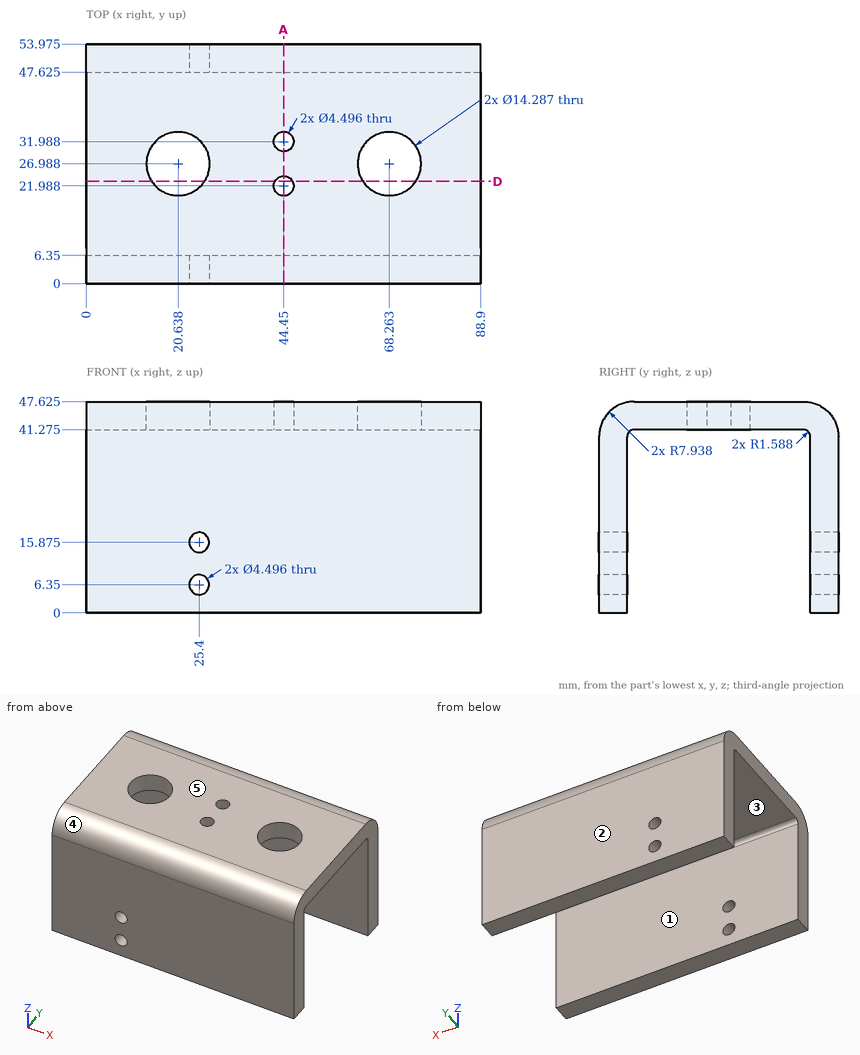
The drawing under review shows one solid part. Ordinate dimensions are in mm from its lowest x, y, z. A direction names the side the tool comes from. Give positions to 0.01 mm unless a question says otherwise; leave off trailing zeros. Write each loop counter-clockwise with the first axis right and the second up, starting at its lowest first coordinate (ties: lowest second). Pieces come first, ordered by that corner, then holes. Notation, with made-up numbers: M -5,71 L 46,71 A23 ccw 46,88 Z; hole C -10,21 d2. An arc over 180 degrees is marked long. Write each question's results on one line, items separated by ' | '. Start each with the question number.
1. Mouldability with a two-part tool opening along Y and no side actions: class the marked faces 3, 4 and 5 as released by +Y, released by -Y, zero draft, split by the parting line, or undercut.
2. We need section D-D (y = 23). Write out the cut boundary in (x, z) (1 decimal).
3. For the marked faces 1 and 2, list the 3-axis set-ups (+Z, -Z, +X, -X, +Y, -Y) from which the entire face can be reached by the end or side of a thin tool; tool diameter is ignored.
4. For probe 1 along Z at (x, y) = (25.4, 1.75) (1 decimal); probe 2 along Z at (x, y) = (25.4, 52.5) (1 decimal); probe 3 along Z at (x, y) = (9, 38.5) (1 decimal), list the stretches that pass through material, from the lowest coordinate up. Write a range as [from, to].
5. We need section A-A (x = 44.45). Count the separate pieces of the cut face and the enclosed holes in it, and give its area (3 significant figures).
6. Insertion check: pin 1 Ø2 at (x, y) = (26.5, 11.5) entering from -Z (1 decimal). The pin has a flat end and moves straight along its axis. Give the tip position at first contact, or say it passes through.
Results found:
1) face 3: undercut | face 4: released by -Y | face 5: zero draft
2) outline: M 0,41.3 L 14.7,41.3 L 14.7,47.6 L 0,47.6 Z; M 26.6,41.3 L 42.4,41.3 L 42.4,47.6 L 26.6,47.6 Z; M 46.5,41.3 L 62.3,41.3 L 62.3,47.6 L 46.5,47.6 Z; M 74.2,41.3 L 88.9,41.3 L 88.9,47.6 L 74.2,47.6 Z
3) face 1: -Z, +X, -X | face 2: +Z, -Z, +X, -X, +Y
4) probe 1: z = [0, 4.1], [8.6, 13.6], [18.1, 44.7] | probe 2: z = [0, 4.1], [8.6, 13.6], [18.1, 44.3] | probe 3: z = [41.3, 47.6]
5) separate pieces: 3 | enclosed holes: 0 | area: 784 mm^2
6) pin 1: stops at z = 41.3
